The listing builds one solid part. Answer for the finished solid, in the listing's coordinates (mm). A direction names the side the tool comes from. Coordinates: 2 decimals unless noted, no trailing zeros. Write each loop counter-clockwise with the first axis right and the second up, starting at its lowest first coordinate (ties: lowest second). Pieces come first, ordered by that corner, then holes.
from build123d import *

# Parameters (mm, degrees)
EXTRUDE_1_DEPTH     = 60
EXTRUDE_2_DEPTH     = 9
SKETCH_7_R          = 11
EXTRUDE_3_DEPTH     = 2
SKETCH_8_R          = 2.5
EXTRUDE_4_DEPTH     = 18
CUT_EXTRUDE_START   = -15
CUT_EXTRUDE_1_DEPTH = 15
SKETCH_10_R         = 1.6
CUT_EXTRUDE_2_DEPTH = 4.5


with BuildPart() as part:
    # 草图2 → 凸台-拉伸1 (new body)
    with BuildSketch(Plane(origin=(0, 0, 0), x_dir=(1, 0, 0), z_dir=(0, 1, 0))):
        Polygon((-14.012734328, 22.447763171), (-21.08380214, 15.376695359), (-21.08380214, -12.681169017), (-14.012734328, -19.752236829), (14.045130048, -19.752236829), (21.11619786, -12.681169017), (21.11619786, 15.376695359), (14.045130048, 22.447763171), align=None)
    extrude(amount=EXTRUDE_1_DEPTH)

    # 草图5 → 凸台-拉伸2 (add)
    with BuildSketch(Plane(origin=(0, 60, 0), x_dir=(1, 0, 0), z_dir=(0, 1, 0))):
        with BuildLine():
            Line((-16.776242784, 22.447763171), (16.776242784, 22.447763171))
            ThreePointArc((16.776242784, 22.447763171), (19.070321818, 20.399669839), (21.11619786, 18.103613191))
            Line((21.11619786, 18.103613191), (21.11619786, -15.408086849))
            ThreePointArc((21.11619786, -15.408086849), (19.070321818, -17.704143498), (16.776242784, -19.752236829))
            Line((16.776242784, -19.752236829), (-16.776242784, -19.752236829))
            ThreePointArc((-16.776242784, -19.752236829), (-19.051917848, -17.722547478), (-21.08380214, -15.448831998))
            Line((-21.08380214, -15.448831998), (-21.08380214, 18.14435834))
            ThreePointArc((-21.08380214, 18.14435834), (-19.051917848, 20.41807382), (-16.776242784, 22.447763171))
        make_face()
    extrude_2 = extrude(amount=-EXTRUDE_2_DEPTH)

    # 镜向1: 凸台-拉伸2 across plane
    add(extrude_2.mirror(Plane.ZX.offset(30)))

    # 草图7 → 凸台-拉伸3 (add)
    with BuildSketch(Plane(origin=(0, 60, 0), x_dir=(1, 0, 0), z_dir=(0, 1, 0))):
        with Locations(Location((0, 1.347763171, 0), (0, 0, 270))):
            Circle(SKETCH_7_R)
    extrude(amount=EXTRUDE_3_DEPTH)

    # 草图8 → 凸台-拉伸4 (add)
    with BuildSketch(Plane(origin=(0, 62, 0), x_dir=(1, 0, 0), z_dir=(0, 1, 0))):
        with Locations(Location((0, 1.347763171, 0), (0, 0, 270))):
            Circle(SKETCH_8_R)
    extrude(amount=EXTRUDE_4_DEPTH)

    # 草图9 → 切除-拉伸1 (cut)
    with BuildSketch(Plane(origin=(0, 80, 0), x_dir=(1, 0, 0), z_dir=(0, 1, 0)).offset(CUT_EXTRUDE_START)):
        with BuildLine():
            Line((-1.785357107, 3.097763171), (1.785357107, 3.097763171))
            ThreePointArc((1.785357107, 3.097763171), (0, 3.847763171), (-1.785357107, 3.097763171))
        make_face()
    extrude(amount=CUT_EXTRUDE_1_DEPTH, mode=Mode.SUBTRACT)

    # 草图10 → 切除-拉伸2 (cut)
    with BuildSketch(Plane(origin=(0, 60, 0), x_dir=(1, 0, 0), z_dir=(0, 1, 0))):
        with Locations(Location((-15.5, 16.847763171, 0), (0, 0, 270))):
            Circle(SKETCH_10_R)
        with Locations(Location((15.5, 16.847763171, 0), (0, 0, 270))):
            Circle(SKETCH_10_R)
        with Locations(Location((15.5, -14.152236829, 0), (0, 0, 270))):
            Circle(SKETCH_10_R)
        with Locations(Location((-15.5, -14.152236829, 0), (0, 0, 270))):
            Circle(SKETCH_10_R)
    extrude(amount=-CUT_EXTRUDE_2_DEPTH, mode=Mode.SUBTRACT)


solid = part.part
Q1. Determine the mould class of faces 1 (the face through (16, 55.5, 14)), 2 (the face through (0, 30, -22.448)), 3 (the face through (17.5, 29.7, 16.3)), 4 (the face through (0, 80, -1)) for opening direction Z: released by +Z, released by -Z, zero draft, split by the parting line, or undercut.
Answers below:
face 1: undercut
face 2: released by -Z
face 3: released by +Z
face 4: zero draft
Q2. The part is cut by section D-D, the plane y = 32.5. Write down the section's boundary in (x, z), then the cut area to 3 significant figures.
Answers below:
outline: (-21.08, -15.38) - (-14.01, -22.45) - (14.05, -22.45) - (21.12, -15.38) - (21.12, 12.68) - (14.05, 19.75) - (-14.01, 19.75) - (-21.08, 12.68) - close
area: 1,680 mm2
Q3. The part is cut by section A-A, the plane x = 0. Write down the section's boundary in (y, z), then the cut area to 3 significant figures.
Answers below:
outline: (0, -22.45) - (60, -22.45) - (60, -12.35) - (62, -12.35) - (62, -3.85) - (65, -3.85) - (65, -3.1) - (80, -3.1) - (80, 1.15) - (62, 1.15) - (62, 9.65) - (60, 9.65) - (60, 19.75) - (0, 19.75) - close
area: 2,650 mm2
Q4. Find the intervals of material crossed by probe 1 along Z at (x, y) = (-15, 58); probe 2 along Y at (x, z) = (-15.5, 17.5); probe 3 along Y at (x, z) = (10, 1), in increasing order.
Answers below:
probe 1: z = -22.45 to -18.37, -15.33 to 12.63, 15.67 to 19.75
probe 2: y = 0 to 60
probe 3: y = 0 to 62
Q5. The part is cut by section C-C, the plane z = -0.5. Write down the section's boundary in (x, y), then the cut area to 3 significant figures.
Answers below:
outline: (-21.08, 0) - (21.12, 0) - (21.12, 60) - (10.97, 60) - (10.97, 62) - (2.35, 62) - (2.35, 80) - (-2.35, 80) - (-2.35, 62) - (-10.97, 62) - (-10.97, 60) - (-21.08, 60) - close
area: 2,660 mm2
Q6. Which of the six approach directions +Z, -Z, +X, -X, +Y, -Y give full straight-line access (tool end or side, diameter ignored) to faces 5 (the face through (-14.42, 57.78, 12.97)), 6 (the face through (18, 51, -20)), 7 (the face through (0, 72, -3.098)), 8 (the face through (-17.598, 29.706, 16.167))?
Answers below:
face 5: +Y
face 6: -Z, +X
face 7: -Z, +X, -X, +Y
face 8: +Z, -X
Q7. Given pin 1 (5 mm diameter, centred on x = 15.5, z = -16.85, fed in from -Y); pin 2 (10 mm diameter, centred on x = 2.5, z = -9.5, fed in from +Y); pin 3 (8 mm diameter, centred on x = 17, z = -19, fed in from +Y); pin 4 (0.6 mm diameter, centred on x = -1, z = -3.5, fed in from +Y), each flat-ended and moving along its own axis, determine where each tip first touches the part or whether it passes through.
Answers below:
pin 1: stops at y = 0
pin 2: stops at y = 62
pin 3: stops at y = 60
pin 4: stops at y = 65
Q8. The part is cut by section B-B, the plane y = 54. Write down the section's boundary in (x, z).
Answers below:
outline: (-21.08, -18.14) arc R26.96 ccw to (-16.78, -22.45) - (16.78, -22.45) arc R26.96 ccw to (21.12, -18.1) - (21.12, 15.41) arc R26.96 ccw to (16.78, 19.75) - (-16.78, 19.75) arc R26.96 ccw to (-21.08, 15.45) - close
